Job drawing, mm, ordinate dimensions from the low corner. One solid piece. Round coordinates to 2 decimals unless told otherwise and drop trailing zeros. Order: outer loops, then holes, each group sorted by start corner. A loop starts at its lowest first (then second) coordinate and runs counter-clockwise, first axis right, second up. Notation, with made-up numbers: (-5, 82) - (41, 82) arc R6 ccw to (41, 91) - close; hole circle Ø11 at (-1.5, 77.25). An arc over 180 degrees is marked (long way). Use one line per item in the form item = value. Start each with the question number.
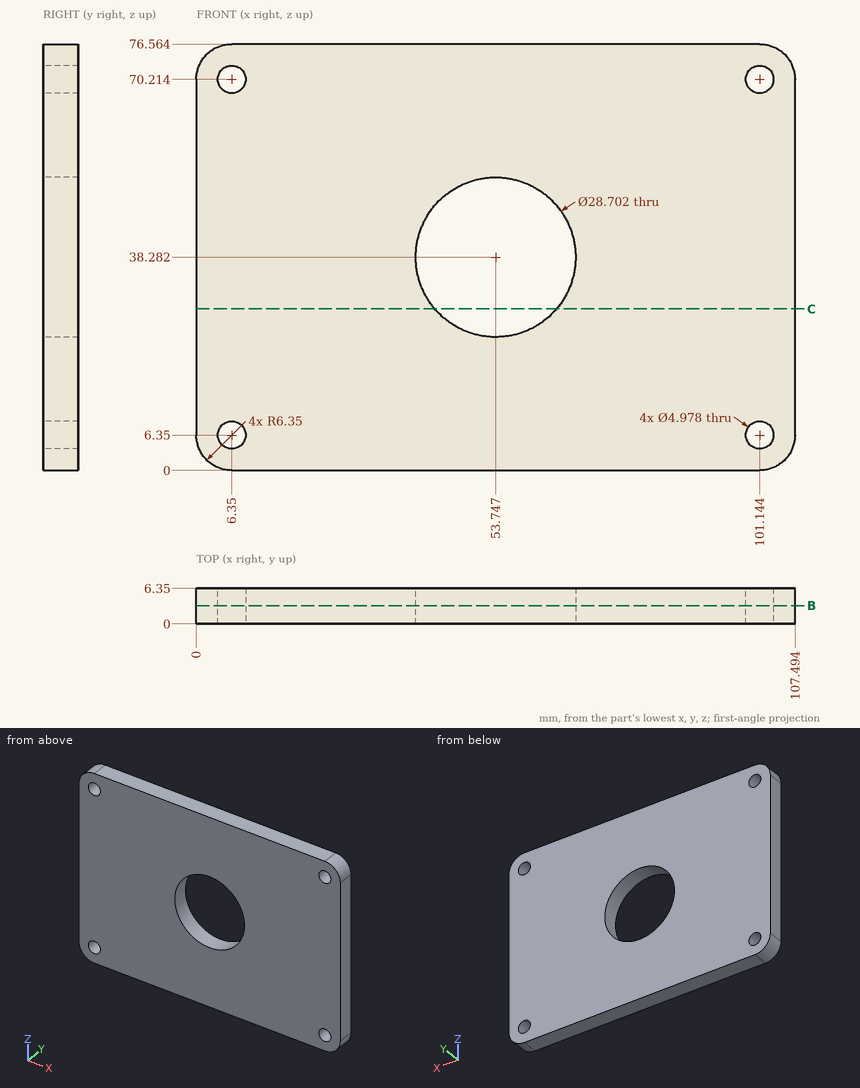
(1) Slice it at B-B (y = 3.25). Give the number of separate pieces and of enclosed holes in the cut face, and give its area (3 significant figures).
(2) Wall check: line 1 (X direction, y = 2, z = 6) (1 decimal); line 2 (Z direction, x = 5.5, y = 5) (1 decimal); line 3 (Z direction, x = 42.5, y = 6) (1 decimal). Give the ranges that are in metal, low to high. Write a range as [from, to].
(3) Flat gauge pin, fed straight in: P1, Ø3, axis at x = 6.35, z = 70.21, coming from the +Y side. Where does the tip first touch, or does it go through?
(4) Slice it at C-C (z = 29). Give the cut face in (x, y).
Results list:
q1.separate_pieces = 1
q1.enclosed_holes = 5
q1.area = 7,470 mm²
q2.line_1 = [0, 3.9], [8.8, 98.7], [103.6, 107.5]
q2.line_2 = [0.1, 4], [8.7, 67.9], [72.6, 76.5]
q2.line_3 = [0, 29.4], [47.2, 76.6]
q3.P1 = through
q4.outline = (0, 0) - (42.8, 0) - (42.8, 6.35) - (0, 6.35) - close; (64.69, 0) - (107.49, 0) - (107.49, 6.35) - (64.69, 6.35) - close
